Check sheet for the modelled part. Datum: model origin and axes. Units: mm. A direction names the side the tool comes from. Give positions to 0.01 mm unless a question says otherwise; leave off trailing zeros. Loops run counter-clockwise (first coordinate to the right, second up) from the corner with the lowest first, then second, coordinate; pieces in that order, holes last. Notation, with made-up numbers: M 32,31.5 L 58,31.5 A18 ccw 58,37.5 Z; hole C 59.25,39.5 d9. An arc over 180 degrees is marked long. Write each question's results on one line, items separated by ' | '. Start each with the question number.
1. Tool access check on faces 4 (the flat face through (69, -12.7, 45)), 5 (the flat face through (22.225, -8, 18)), 6 (the flat face through (103.794, 0, 64)). Record the directions out of +Z, -Z, +X, -X, +Y, -Y that give a thin tool (end or side, any length) a straight path to the whole face; none if there is none.
2. Sectioned sample at A-A on y = 40. Record the cut outline in (x, z) (3 decimals).
3. Sectioned sample at B-B on x = 96. Record the cut outline in (y, z).
4. Draft check along X on faces 1 (the cylindrical face through (30.741, 7.871, 49.855)), 2 (the cylindrical face through (45.8, -0.2, 38.1)), 3 (the flat face through (-1, 63.5, 0)). Enter one of: pulls with the +X half, pulls with the -X half, needs draft (parallel to the pull), parting line crosses it, or undercut.
5. Go/stop test with flat-tipped pins: pin 1 (4 mm diameter, centred on x = 76, z = 54, fed in from -Y); pin 2 (10 mm diameter, centred on y = 6.5, z = 36.5, fed in from +X) (3 decimals); pin 3 (5 mm diameter, centred on y = 7.5, z = 17, fed in from -X) (3 decimals); pin 4 (17 mm diameter, centred on x = 85, z = 39.5, fed in from +Y). Record where each tip stops, or that it passes through.
6. Material ranges on line 1 along X through (y, z) = (34.5, -6) (3 decimals); line 2 along Z through (x, y) = (-28.5, 12) (3 decimals); line 3 along Y through (x, z) = (101.5, 43.5), recorded low to high.
```python
from build123d import *

# Parameters (mm, degrees)
F1_DEPTH = 63.5
F0_W     = 38.4694138315
F0_H     = 19.05
F2_DEPTH = 12.7
F3_DEPTH = 3.175


with BuildPart() as f1:
    # F0 (on Front) → F1 (new body, symmetric)
    with BuildSketch(Plane.XZ):
        Polygon((-41.275, -9.525), (41.275, -9.525), (41.275, 9.525), (22.225, 9.525), (-41.275, 9.525), align=None)
    extrude(amount=F1_DEPTH, both=True)

    # F0 (on Front) → F2 (join, symmetric)
    with BuildSketch(Plane.XZ):
        with BuildLine():
            Line((22.225, 9.525), (41.275, 9.525))
            Line((41.275, 9.525), (41.275, 27.0002))
            ThreePointArc((41.275, 27.0002), (45.9246798487, 38.2255201513), (57.15, 42.8752))
            Line((57.15, 42.8752), (65.3250142932, 42.8752))
            Line((65.3250142932, 42.8752), (65.3250142932, 61.9252))
            Line((65.3250142932, 61.9252), (57.15, 61.9252))
            add(Edge.make_bspline(
                [(51.4572367621, 61.4581174025), (53.3370613896, 61.6402112434), (55.2348987126, 61.7960082111), (57.15, 61.9252)],
                knots=[106.9298065105, 106.9298065105, 106.9298065105, 106.9298065105, 111.5045361635, 111.5045361635, 111.5045361635, 111.5045361635], degree=3))
            ThreePointArc((51.4572367621, 61.4581174025), (30.517544414, 49.593737449), (22.225, 27.0002))
            Line((22.225, 27.0002), (22.225, 9.525))
        make_face()
        Polygon((103.7944281247, 61.9252), (103.7944281247, 42.8752), (103.7944281247, 38.1), (116.1250142932, 38.1), (116.1250142932, 66.675), (103.7944281247, 66.675), align=None)
        with Locations((84.559721209, 52.4002)):
            Rectangle(F0_W, F0_H)
    extrude(amount=F2_DEPTH, both=True)

    # F0 (on Front) → F3 (join, symmetric)
    with BuildSketch(Plane.XZ):
        with BuildLine():
            add(Edge.make_bspline(
                [(-41.275, 9.525), (-26.5797272303, 38.5784325229), (7.5181848531, 57.2018529553), (51.4572367621, 61.4581174025)],
                knots=[0, 0, 0, 0, 106.9298065105, 106.9298065105, 106.9298065105, 106.9298065105], degree=3))
            Line((-41.275, 9.525), (22.225, 9.525))
            Line((22.225, 9.525), (22.225, 27.0002))
            ThreePointArc((22.225, 27.0002), (30.517544414, 49.593737449), (51.4572367621, 61.4581174025))
        make_face()
    extrude(amount=F3_DEPTH, both=True)


solid = f1.part
```
Output values:
1) face 4: +Z, +X, -X, -Y | face 5: +Z, -X, -Y | face 6: +Z, -X, +Y, -Y
2) outline: M -41.275,-9.525 L 41.275,-9.525 L 41.275,9.525 L -41.275,9.525 Z
3) outline: M -12.7,42.88 L 12.7,42.88 L 12.7,61.93 L -12.7,61.93 Z
4) face 1: pulls with the -X half | face 2: undercut | face 3: needs draft
5) pin 1: y = -12.7 | pin 2: x = 116.125 | pin 3: x = 22.225 | pin 4: y = 12.7
6) line 1: -41.275 to 41.275 | line 2: -9.525 to 9.525 | line 3: -12.7 to 12.7
